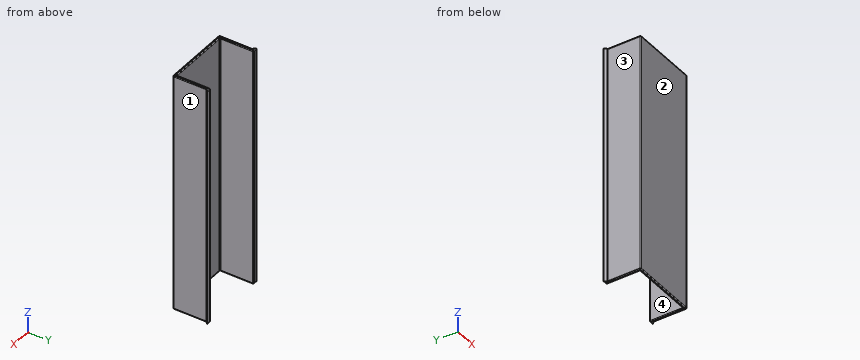
```python
from build123d import *

# Parameters (mm, degrees)
F1_DEPTH = 150
F2_R     = 0.5


with BuildPart() as f1:
    # F0 (on Top) → F1 (new body)
    with BuildSketch(Plane.XY):
        Polygon((-41.5, 1.5), (-41.5, 22.562249), (-44.5, 22.562249), (-43, 21.062249), (-43, 0), (0, 0), (0, 21.062249), (1.5, 22.562249), (-1.5, 22.562249), (-1.5, 1.5), align=None)
    extrude(amount=F1_DEPTH)

    # F2
    f2_edges = [f1.edges().sort_by_distance(p)[0] for p in [
        (-1.5, 22.562249, 75),
        (-1.5, 12.031124, 150),
        (-1.5, 1.5, 75),
        (0, 10.531124, 150),
        (-21.5, 0, 150),
        (-41.5, 12.031124, 150),
        (-41.5, 22.562249, 75),
        (-21.5, 1.5, 0),
        (-21.5, 1.5, 150),
        (-41.5, 1.5, 75),
        (0, 0, 75),
        (-21.5, 0, 0),
        (0, 10.531124, 0),
        (-43, 0, 75),
        (-43, 10.531124, 150),
        (-43, 10.531124, 0),
        (-41.5, 12.031124, 0),
        (-1.5, 12.031124, 0),
        (-43, 22.562249, 150),
        (0, 22.562249, 150),
        (0, 22.562249, 0),
        (-43, 22.562249, 0),
    ]]
    fillet(f2_edges, radius=F2_R)


solid = f1.part
```
Input: part model. Units: mm. Frame: model coordinates. Face numbers are marked on the shaded views. Give positions to 0.01 mm unless a question says otherwise; leave off trailing zeros. Write each loop counter-clockwise with the first axis right and the second up, starting at its lowest first coordinate (ties: lowest second). Pieces come first, ordered by that corner, then holes. Notation, with made-up numbers: (61.5, 63) - (76.5, 63) arc R14 ccw to (76.5, 74) - close; hole circle Ø6 at (31, 24). An arc over 180 degrees is marked (long way). Write item = value, one per line. Start each with the question number.
1) Material intervals for L1, parallel to X at y = 9, z = 38; L2, parallel to Y at x = -7, z = 74, sorted ascending. Write a range as [from, to].
2) Cut plane B-B (x = -25). Return loops of the section in (y, z), and give its area (3 significant figures).
3) Cut plane A-A (y = 10). Return loops of the section in (x, z).
4) Pin query (flat end, axial travel): pin 1 (2 mm diameter, centred on y = 13, z = 91, fed in from +X); pin 2 (4 mm diameter, centred on x = -18.5, z = 50, fed in from +Y). Return the tip coordinate at first contact, or that it passes through.
5) Cut plane C-C (z = 39). Return loops of the section in (x, y), and give its area (3 significant figures).
6) Draft query along X for the marked faces 1, 2, 3 and 4. Return one class per face: pulls with the +X half, pulls with the -X half, needs draft (parallel to the pull), parting line crosses it, or undercut.
Answers follow:
q1.L1 = [-43, -41.5], [-1.5, 0]
q1.L2 = [0, 1.5]
q2.outline = (0, 0.5) arc R0.5 ccw to (0.5, 0) - (1, 0) arc R0.5 ccw to (1.5, 0.5) - (1.5, 149.5) arc R0.5 ccw to (1, 150) - (0.5, 150) arc R0.5 ccw to (0, 149.5) - close
q2.area = 225 mm^2
q3.outline = (-43, 0.5) arc R0.5 ccw to (-42.5, 0) - (-42, 0) arc R0.5 ccw to (-41.5, 0.5) - (-41.5, 149.5) arc R0.5 ccw to (-42, 150) - (-42.5, 150) arc R0.5 ccw to (-43, 149.5) - close; (-1.5, 0.5) arc R0.5 ccw to (-1, 0) - (-0.5, 0) arc R0.5 ccw to (0, 0.5) - (0, 149.5) arc R0.5 ccw to (-0.5, 150) - (-1, 150) arc R0.5 ccw to (-1.5, 149.5) - close
q4.pin_1 = 0
q4.pin_2 = 1.5
q5.outline = (-44.5, 22.56) - (-43, 21.06) - (-43, 0.5) arc R0.5 ccw to (-42.5, 0) - (-0.5, 0) arc R0.5 ccw to (0, 0.5) - (0, 21.06) - (1.5, 22.56) - (-1, 22.56) arc R0.5 ccw to (-1.5, 22.06) - (-1.5, 2) arc R0.5 cw to (-2, 1.5) - (-41, 1.5) arc R0.5 cw to (-41.5, 2) - (-41.5, 22.06) arc R0.5 ccw to (-42, 22.56) - close
q5.area = 130 mm^2
q6.face_1 = pulls with the +X half
q6.face_2 = needs draft
q6.face_3 = pulls with the -X half
q6.face_4 = undercut
